```python
from build123d import *

# Parameters (mm, degrees)
BOSS_EXTRUDE1_DEPTH = 8.6
BOSS_EXTRUDE2_DEPTH = 3
SKETCH3_R           = 2
BOSS_EXTRUDE3_DEPTH = 2.75
CUT_EXTRUDE1_REACH  = 25.477
SKETCH4_R           = 1
CHAMFER1_SIZE       = 1.5


with BuildPart() as part:
    # Sketch1 → Boss-Extrude1 (new body)
    with BuildSketch(Plane(origin=(0, 0, 0), x_dir=(0, 0, -1), z_dir=(1, 0, 0))):
        Polygon((9.85, -3.75), (14.6, -3.75), (14.6, -4.75), (9.85, -4.75), (9.85, -20), (-9.85, -20), (-9.85, -4.75), (-14.6, -4.75), (-14.6, -3.75), (-9.85, -3.75), (-9.85, 0), (9.85, 0), align=None)
    extrude(amount=BOSS_EXTRUDE1_DEPTH)

    # Sketch2 → Boss-Extrude2 (add)
    with BuildSketch(Plane(origin=(0, 0, 0), x_dir=(1, 0, 0), z_dir=(0, 1, 0))):
        with BuildLine():
            ThreePointArc((1.907962607, -1.976744186), (4.3, -9.85), (6.692037393, -1.976744186))
            ThreePointArc((6.692037393, -1.976744186), (4.3, 1.25), (1.907962607, -1.976744186))
        make_face()
    extrude(amount=BOSS_EXTRUDE2_DEPTH)

    # Sketch3 → Boss-Extrude3 (add)
    with BuildSketch(Plane(origin=(0, 3, 0), x_dir=(1, 0, 0), z_dir=(0, 1, 0))):
        with Locations(Location((4.3, -5.55, 0), (0, 0, 270))):
            Circle(SKETCH3_R)
    extrude(amount=BOSS_EXTRUDE3_DEPTH)

    # Sketch4 → Cut-Extrude1 (cut, up to next)
    with BuildSketch(Plane(origin=(0, -3.75, 0), x_dir=(1, 0, 0), z_dir=(0, 1, 0)), mode=Mode.PRIVATE) as cut_extrude1_sk1:
        with Locations(Location((4.3, -12.6, 0), (0, 0, 270))):
            Circle(SKETCH4_R)
    cut_extrude1_tool1 = extrude(cut_extrude1_sk1.sketch, amount=-CUT_EXTRUDE1_REACH, mode=Mode.PRIVATE) & part.part
    cut_extrude1 = cut_extrude1_tool1.solids().sort_by_distance((4.3, -3.75, 12.6))[0]
    add(cut_extrude1, mode=Mode.SUBTRACT)

    # Mirror1: Cut-Extrude1 across plane
    add(cut_extrude1.mirror(Plane.XY), mode=Mode.SUBTRACT)

    # Chamfer1
    chamfer1_edges = [part.edges().sort_by_distance(p)[0] for p in [
        (8.6, -4.25, 14.6),
        (0, -4.25, -14.6),
        (0, -4.25, 14.6),
        (8.6, -4.25, -14.6),
    ]]
    chamfer(chamfer1_edges, length=CHAMFER1_SIZE)


solid = part.part
```
Geometry: final body of the model. Coordinates: model frame, mm. A direction names the side the tool comes from. Round coordinates to 2 decimals unless told otherwise and drop trailing zeros. Order: outer loops, then holes, each group sorted by start corner. A loop starts at its lowest first (then second) coordinate and runs counter-clockwise, first axis right, second up. Notation, with made-up numbers: (83, -23) - (137, -23) arc R20 cw to (137, -16) - close; hole circle Ø3 at (38, -16). An arc over 180 degrees is marked (long way). Write item = value, one per line. Start each with the question number.
Q1. Cut plane B-B on x = 8.25. Return the cut outline in (y, z).
Q2. Cut plane C-C on z = 1.25. Return the cut outline in (x, y).
Q3. Pull-direction query (X, two-part tool) for faces 1 (the flat face through (7.8, -4.2, -13.9)), 2 (the cylindrical face through (4.146, 1.479, 9.847)), 3 (the cylindrical face through (4.6, -4.243, -13.554)); classes: +X half, -X half, draft (parallel to the pull), parting line (faces both ways), or undercut.
Q4. Pin query (flat end, axial travel): pin 1 (4.5 mm diameter, centred on x = 5.5, y = -11.5, fed in from -Z); pin 2 (5 mm diameter, centred on x = 4, z = 12, fed in from -Y); pin 3 (2.5 mm diameter, centred on x = 6, z = 13.5, fed in from +Y); pin 4 (5 mm diameter, centred on x = 6, z = -12, fed in from +Y). Return the tip coordinate at first contact, or that it passes through.
Q5. Ray query, line 1 (X direction, y = -4.05, z = -12.6); line 2 (Y direction, x = 3.5, z = -8.75); line 3 (Z direction, x = 8, y = -7.75). Return the intervals inside material, ascending. Write a range as from..to.
Q6. Cut plane D-D on y = -10. Return the cut outline in (x, z), and give its area (3 significant figures).
Q7. Access query for faces 4 (the flat face through (8, 0, 9)), 5 (the flat face through (4, 3, 3)), 6 (the flat face through (4, -3.75, -11)), 7 (the flat face through (4, -12, 9.85)). Directions: +Z, -Z, +X, -X, +Y, -Y. A direction counts if a zero-diameter tool reaches every point of the face in a straight line with its end or side. Return the directions, or none.
Q8. Cut plane A-A on z = -12.6. Return the cut outline in (x, y), and give its area (3 significant figures).
Outcome:
q1.outline = (-20, -9.85) - (-4.75, -9.85) - (-4.75, -13.45) - (-3.75, -13.45) - (-3.75, -9.85) - (0, -9.85) - (0, 3.85) - (3, 3.85) - (3, 7.25) - (0, 7.25) - (0, 9.85) - (-3.75, 9.85) - (-3.75, 13.45) - (-4.75, 13.45) - (-4.75, 9.85) - (-20, 9.85) - close
q2.outline = (0, -20) - (8.6, -20) - (8.6, 0) - (6.8, 0) - (6.8, 3) - (1.8, 3) - (1.8, 0) - (0, 0) - close
q3.face_1 = +X half
q3.face_2 = parting line
q3.face_3 = undercut
q4.pin_1 = -9.85
q4.pin_2 = -20
q4.pin_3 = -3.75
q4.pin_4 = 0
q5.line_1 = 0..3.3, 5.3..8.6
q5.line_2 = -20..0
q5.line_3 = -9.85..9.85
q6.outline = (0, -9.85) - (8.6, -9.85) - (8.6, 9.85) - (0, 9.85) - close
q6.area = 169 mm^2
q7.face_4 = +Z, +X, +Y
q7.face_5 = +Y
q7.face_6 = -Z, +X, -X, +Y
q7.face_7 = +Z, +X, -X, -Y
q8.outline = (0, -4.75) - (3.3, -4.75) - (3.3, -3.75) - (0, -3.75) - close; (5.3, -4.75) - (8.6, -4.75) - (8.6, -3.75) - (5.3, -3.75) - close
q8.area = 6.60 mm^2
